from build123d import *

# Parameters (mm, degrees)
SKETCH1_W            = 7.5
SKETCH1_H            = 10
BOSS_EXTRUDE1_DEPTH  = 1
BOSS_EXTRUDE2_DEPTH  = 2.5
SKETCH10_W           = 7.5
SKETCH10_H           = 1
BOSS_EXTRUDE5_DEPTH  = 2
SKETCH56_W           = 7.5
SKETCH56_H           = 1
BOSS_EXTRUDE17_DEPTH = 2
SKETCH57_W           = 3
SKETCH57_H           = 1
BOSS_EXTRUDE18_DEPTH = 5
SKETCH58_W           = 1.5
SKETCH58_H           = 1
BOSS_EXTRUDE19_DEPTH = 2
SKETCH59_W           = 1.5
SKETCH59_H           = 1
BOSS_EXTRUDE20_DEPTH = 2
SKETCH60_W           = 1
SKETCH60_H           = 1.5
BOSS_EXTRUDE23_DEPTH = 1.5
SKETCH61_W           = 1
SKETCH61_H           = 0.75
CUT_EXTRUDE1_DEPTH   = 0.5
SKETCH62_W           = 6
SKETCH62_H           = 12
BOSS_EXTRUDE25_DEPTH = 3
SKETCH64_W           = 4
SKETCH64_H           = 2
CUT_EXTRUDE2_DEPTH   = 12
SKETCH65_W           = 4
SKETCH65_H           = 1
BOSS_EXTRUDE26_DEPTH = 3
SKETCH66_R           = 1
CUT_EXTRUDE3_DEPTH   = 1
SKETCH67_W           = 3
SKETCH67_H           = 1
BOSS_EXTRUDE27_DEPTH = 3
SKETCH68_W           = 3
SKETCH68_H           = 1
BOSS_EXTRUDE28_DEPTH = 3


with BuildPart() as part:
    # Sketch1 → Boss-Extrude1 (new body)
    with BuildSketch(Plane(origin=(0, 0, 0), x_dir=(1, 0, 0), z_dir=(0, 1, 0))):
        Rectangle(SKETCH1_W, SKETCH1_H)
    extrude(amount=BOSS_EXTRUDE1_DEPTH)

    # Sketch2 → Boss-Extrude2 (add)
    with BuildSketch(Plane(origin=(0, 1, 0), x_dir=(1, 0, 0), z_dir=(0, 1, 0))):
        Polygon((-3.75, 3), (-2.1, 5), (-3.75, 5), align=None)
        Polygon((3.75, 5), (2.1, 5), (3.75, 3), align=None)
    extrude(amount=BOSS_EXTRUDE2_DEPTH)

    # Sketch10 → Boss-Extrude5 (add)
    with BuildSketch(Plane.XY.offset(5)):
        with Locations((0, 0.5)):
            Rectangle(SKETCH10_W, SKETCH10_H)
    extrude(amount=BOSS_EXTRUDE5_DEPTH)

    # Sketch56 → Boss-Extrude17 (add)
    with BuildSketch(Plane.XY.offset(7)):
        with Locations((0, 0.5)):
            Rectangle(SKETCH56_W, SKETCH56_H)
    extrude(amount=BOSS_EXTRUDE17_DEPTH)

    # Sketch57 → Boss-Extrude18 (add)
    with BuildSketch(Plane(origin=(0, 0, -5), x_dir=(-1, 0, 0), z_dir=(0, 0, -1))):
        with Locations((0, 0.5)):
            Rectangle(SKETCH57_W, SKETCH57_H)
    extrude(amount=BOSS_EXTRUDE18_DEPTH)

    # Sketch58 → Boss-Extrude19 (add)
    with BuildSketch(Plane(origin=(1.5, 0, 0), x_dir=(0, 0, -1), z_dir=(1, 0, 0))):
        with Locations((9.25, 0.5)):
            Rectangle(SKETCH58_W, SKETCH58_H)
    extrude(amount=BOSS_EXTRUDE19_DEPTH)

    # Sketch59 → Boss-Extrude20 (add)
    with BuildSketch(Plane.ZY.offset(1.5)):
        with Locations((-9.25, 0.5)):
            Rectangle(SKETCH59_W, SKETCH59_H)
    extrude(amount=BOSS_EXTRUDE20_DEPTH)

    # Sketch60 → Boss-Extrude23 (add)
    with BuildSketch(Plane(origin=(0, 1, 0), x_dir=(1, 0, 0), z_dir=(0, 1, 0))):
        with Locations((3, 9.25)):
            Rectangle(SKETCH60_W, SKETCH60_H)
        with Locations((-3, 9.25)):
            Rectangle(SKETCH60_W, SKETCH60_H)
    extrude(amount=BOSS_EXTRUDE23_DEPTH)

    # Sketch61 → Cut-Extrude1 (cut)
    with BuildSketch(Plane(origin=(0, 2.5, 0), x_dir=(1, 0, 0), z_dir=(0, 1, 0))):
        with Locations((-3, 9.245443114)):
            Rectangle(SKETCH61_W, SKETCH61_H)
        with Locations((3, 9.245443114)):
            Rectangle(SKETCH61_W, SKETCH61_H)
    extrude(amount=-CUT_EXTRUDE1_DEPTH, mode=Mode.SUBTRACT)

    # Sketch62 → Boss-Extrude25 (add)
    with BuildSketch(Plane(origin=(0, 0, 0), x_dir=(-1, 0, 0), z_dir=(0, -1, 0))):
        with Locations((0, -1)):
            Rectangle(SKETCH62_W, SKETCH62_H)
    extrude(amount=BOSS_EXTRUDE25_DEPTH)

    # Sketch64 → Cut-Extrude2 (cut)
    with BuildSketch(Plane.XY.offset(7)):
        with Locations((0, -1)):
            Rectangle(SKETCH64_W, SKETCH64_H)
    extrude(amount=-CUT_EXTRUDE2_DEPTH, mode=Mode.SUBTRACT)

    # Sketch65 → Boss-Extrude26 (add)
    with BuildSketch(Plane(origin=(0, 0, -5), x_dir=(-1, 0, 0), z_dir=(0, 0, -1))):
        with Locations((0, -2.5)):
            Rectangle(SKETCH65_W, SKETCH65_H)
    extrude(amount=BOSS_EXTRUDE26_DEPTH)

    # Sketch66 → Cut-Extrude3 (cut)
    with BuildSketch(Plane(origin=(0, -3, 0), x_dir=(-1, 0, 0), z_dir=(0, -1, 0))):
        with Locations((0, -5)):
            Circle(SKETCH66_R)
        with Locations((0, 5)):
            Circle(SKETCH66_R)
    extrude(amount=-CUT_EXTRUDE3_DEPTH, mode=Mode.SUBTRACT)

    # Sketch67 → Boss-Extrude27 (add)
    with BuildSketch(Plane.ZY.offset(3)):
        with Locations((-1.5, -1.5)):
            Rectangle(SKETCH67_W, SKETCH67_H)
    extrude(amount=BOSS_EXTRUDE27_DEPTH)

    # Sketch68 → Boss-Extrude28 (add)
    with BuildSketch(Plane(origin=(3, 0, 0), x_dir=(0, 0, -1), z_dir=(1, 0, 0))):
        with Locations((1.5, -1.5)):
            Rectangle(SKETCH68_W, SKETCH68_H)
    extrude(amount=BOSS_EXTRUDE28_DEPTH)


solid = part.part
Geometry: final body of the model. Coordinates: model frame, mm. A direction names the side the tool comes from. Give positions to 0.01 mm unless a question says otherwise; leave off trailing zeros. Write each loop counter-clockwise with the first axis right and the second up, starting at its lowest first coordinate (ties: lowest second). Pieces come first, ordered by that corner, then holes. Notation, with made-up numbers: (45.25, 42.25) - (49.25, 42.25) arc R21 cw to (49.25, 70.25) - close; hole circle Ø11 at (50.25, 74). An arc over 180 degrees is marked (long way). Return JSON: item names as keys, results as strings. Group by question number.
1) First-contact query: P1, Ø2, axis at x = -0.5, z = 4, coming from the +Y side; P2, Ø1, axis at y = 1, z = 4.5, coming from the -X side; P3, Ø3, axis at x = 4, y = -2, coming from the +Z side. Flat tips, straight axial feed; report the tip coordinate or a pass-through.
2) Section B-B on z = 5. Return the cut outline in (x, y).
3) Mould query, pull axis Z, two halves, no side actions, for faces 1 (the flat face through (0, -2.5, 7)), 2 (the flat face through (0, 1, 1)), 3 (the flat face through (-3, 1, -5)). Classes: released by +Z, released by -Z, zero draft, split by the parting line, or undercut.
4) Line query: line 1 (Y direction, x = 0, z = 3.5); line 2 (Z direction, x = 0, y = -2.7); line 3 (X direction, y = -1.5, z = 2.5). Output: solid intervals per line, ascending.
5) Set-up query: faces 4 (the flat face through (2, -2.5, -6.5)), 5 (the cylindrical face through (0.13, -2.51, -5.99)), 6 (the flat face through (-3.5, 1, -9)). Return all of +Z, -Z, +X, -X, +Y, -Y with unobstructed straight access to the full face (end or side cutting, diameter ignored); none if empty.
6) Section D-D on x = 0. Return the cut outline in (y, z), plus the area to 3 significant figures.
7) Section C-C on y = -0.25. Return the cut outline in (x, z).
8) Section A-A on y = 2.25. Return the cut outline in (x, z), plus the area to 3 significant figures.
Filled in:
{
 "1": {"P1": "stops at y = 1", "P2": "stops at x = -3.75", "P3": "stops at z = 7"},
 "2": {"outline": "(-3.75, 0) - (-3, 0) - (-3, -3) - (-1, -3) - (-1, -2) - (-2, -2) - (-2, 0) - (2, 0) - (2, -2) - (1, -2) - (1, -3) - (3, -3) - (3, 0) - (3.75, 0) - (3.75, 1) - (-3.75, 1) - close"},
 "3": {"face 1": "released by +Z", "face 2": "zero draft", "face 3": "undercut"},
 "4": {"line 1": "y = -3 to -2, 0 to 1", "line 2": "z = -8 to -6, -4 to 4, 6 to 7", "line 3": "x = -3 to -2, 2 to 3"},
 "5": {"face 4": "-Z, +X, +Y, -Y", "face 5": "-Y", "face 6": "-Z, -X, +Y, -Y"},
 "6": {"outline": "(-3, -8) - (-2, -8) - (-2, -6) - (-3, -6) - close; (-3, -4) - (-2, -4) - (-2, 4) - (-3, 4) - close; (-3, 6) - (-2, 6) - (-2, 7) - (-3, 7) - close; (0, -10) - (1, -10) - (1, 9) - (0, 9) - close", "area": "30.0 mm^2"},
 "7": {"outline": "(-3, -5) - (-2, -5) - (-2, 7) - (-3, 7) - close; (2, -5) - (3, -5) - (3, 7) - (2, 7) - close"},
 "8": {"outline": "(-3.75, -5) - (-2.1, -5) - (-3.75, -3) - close; (-3.5, -10) - (-2.5, -10) - (-2.5, -9.62) - (-3.5, -9.62) - close; (-3.5, -8.87) - (-2.5, -8.87) - (-2.5, -8.5) - (-3.5, -8.5) - close; (2.1, -5) - (3.75, -5) - (3.75, -3) - close; (2.5, -10) - (3.5, -10) - (3.5, -9.62) - (2.5, -9.62) - close; (2.5, -8.87) - (3.5, -8.87) - (3.5, -8.5) - (2.5, -8.5) - close", "area": "4.80 mm^2"}
}
